Autodesk Inventor part; units mm, degrees
ref_plane "YZ Plane" through (0, 0, 0) normal (1, 0, 0) x (0, 1, 0)
ref_plane "XZ Plane" through (0, 0, 0) normal (0, 1, 0) x (-1, 0, 0)
ref_plane "XY Plane" through (0, 0, 0) normal (0, 0, 1) x (1, 0, 0)
sketch "Эскиз1" plane through (0, 0, 0) normal (1, 0, 0) x (0, 1, 0)
  line L0 (0, -5.7735) -> (-5, -2.8868)
  line L1 (-5, -2.8868) -> (-5, 2.8868)
  line L2 (-5, 2.8868) -> (0, 5.7735)
  line L3 (0, 5.7735) -> (5, 2.8868)
  line L4 (5, 2.8868) -> (5, -2.8868)
  line L5 (5, -2.8868) -> (0, -5.7735)
  circle A0 centre (0, 0) radius 3
  dimension "d0" = 10
  dimension "d1" = 6
extrude "Выдавливание1" add sketch "Эскиз1" along normal blind 5
chamfer "Фаска1" distance 0.5 angle 45 12 edges at (5, 2.5, 4.3301) (5, 5, 0) (5, 2.5, -4.3301) (5, -2.5, -4.3301) (5, -5, 0) (5, -2.5, 4.3301) (0, 2.5, 4.3301) (0, -2.5, 4.3301) (0, 5, 0) (0, 2.5, -4.3301) (0, -2.5, -4.3301) (0, -5, 0)
properties part number "04-01-Гайка М10"
Work out the finished part from the listing and answer in its coordinate system (mm). Give positions to 0.01 mm unless a question says otherwise; leave off trailing zeros. Order: outer loops, then holes, each group sorted by start corner. A loop starts at its lowest first (then second) coordinate and runs counter-clockwise, first axis right, second up.
1. The mould has two halves that part along Y. Classify faces 1 (the cylindrical face through (2, -3, 0)), 2 (the flat face through (2, -5, 0)), 3 (the flat face through (2.472, 2.465, 4.35)): released by +Y, released by -Y, zero draft, split by the parting line, or undercut.
Result sheet:
face 1: undercut
face 2: released by -Y
face 3: released by +Y
2. Section C-C, the plane y = -1.25 is taken. Determine the outline of the cut face in (x, z).
Result sheet:
outline: (0, -4.47) - (0.5, -5.05) - (4.5, -5.05) - (5, -4.47) - (5, -2.73) - (0, -2.73) - close; (0, 2.73) - (5, 2.73) - (5, 4.47) - (4.5, 5.05) - (0.5, 5.05) - (0, 4.47) - close
3. Section B-B, the plane x = 1.55 is taken. Determine the outline of the cut face in (y, z).
Result sheet:
outline: (-5, -2.89) - (0, -5.77) - (5, -2.89) - (5, 2.89) - (0, 5.77) - (-5, 2.89) - close; hole circle Ø6 at (0, 0)
4. Section D-D, the plane y = -3.75 is taken. Determine the outline of the cut face in (x, z).
Result sheet:
outline: (0, -3.03) - (0.5, -3.61) - (4.5, -3.61) - (5, -3.03) - (5, 3.03) - (4.5, 3.61) - (0.5, 3.61) - (0, 3.03) - close
5. This flat-tipped pin is pushed along its axis until it touches: P1, Ø1.5, axis at x = 3, y = -1, coming from the -Z side. Where does it stop, or does it pass through?
Result sheet:
P1: stops at z = -5.63
6. Straight lines are drawn through the part: L1, parallel to Z at x = 2.9, y = -2.5; L2, parallel to Y at x = 3.4, z = 2.25; L3, parallel to Y at x = 2.65, z = 1. For each, find the intervals that lie inside material, in ascending order.
Result sheet:
L1: z = -4.33 to -1.66, 1.66 to 4.33
L2: y = -5 to -1.98, 1.98 to 5
L3: y = -5 to -2.83, 2.83 to 5
7. Section A-A, the plane z = 0 is taken. Determine the outline of the cut face in (x, y), and give its area (3 significant figures).
Result sheet:
outline: (0, -4.5) - (0.5, -5) - (4.5, -5) - (5, -4.5) - (5, -3) - (0, -3) - close; (0, 3) - (5, 3) - (5, 4.5) - (4.5, 5) - (0.5, 5) - (0, 4.5) - close
area: 19.5 mm2
